Geometry: final body of the model. Coordinates: model frame, mm. Give positions to 0.01 mm unless a question says otherwise; leave off trailing zeros. Loops run counter-clockwise (first coordinate to the right, second up) from the corner with the lowest first, then second, coordinate; pieces in that order, holes last. Notation, with made-up numbers: (27, 72) -> (56, 72) arc R11 cw to (56, 93) -> close; hole circle Ø4 at (60, 57). An arc over 180 degrees is marked (long way). One line per item, written item: value. Start each with the question number.
from build123d import *
from OCP.BRepFilletAPI import BRepFilletAPI_MakeChamfer

# Parameters (mm, degrees)
BOSS_EXTRUDE1_DEPTH = 6
SKETCH2_W           = 9.8
SKETCH2_H           = 5.8
CUT_EXTRUDE1_DEPTH  = 6
SKETCH5_W           = 20
SKETCH5_H           = 236
CUT_EXTRUDE2_DEPTH  = 6
SKETCH6_W           = 10
SKETCH6_H           = 204
CUT_EXTRUDE3_DEPTH  = 20
SKETCH7_W           = 32
SKETCH7_H           = 236
CUT_EXTRUDE4_DEPTH  = 20
SKETCH8_W           = 248
SKETCH8_H           = 6
BOSS_EXTRUDE2_DEPTH = 5
SKETCH10_W          = 30
SKETCH10_H          = 204
BOSS_EXTRUDE3_DEPTH = 6
SKETCH11_W          = 21
SKETCH11_H          = 6
BOSS_EXTRUDE4_DEPTH = 30
CHAMFER1_SIZE       = 30
CHAMFER1_SIZE2      = 10.919107028
FILLET1_R           = 10


with BuildPart() as part:
    # Sketch1 → Boss-Extrude1 (new body)
    with BuildSketch(Plane(origin=(0, 0, 0), x_dir=(1, 0, 0), z_dir=(0, 1, 0))):
        Polygon((-150, 118), (-150, -118), (150, -118), (150, -102), (-98, -102), (-98, 102), (150, 102), (150, 118), align=None)
    extrude(amount=BOSS_EXTRUDE1_DEPTH)

    # Sketch2 → Cut-Extrude1 (cut)
    with BuildSketch(Plane(origin=(0, 6, 0), x_dir=(1, 0, 0), z_dir=(0, 1, 0))):
        with Locations((85, -110)):
            Rectangle(SKETCH2_W, SKETCH2_H)
        with Locations((115, -110)):
            Rectangle(SKETCH2_W, SKETCH2_H)
        with Locations((55, -110)):
            Rectangle(SKETCH2_W, SKETCH2_H)
        with Locations((25, -110)):
            Rectangle(SKETCH2_W, SKETCH2_H)
        with Locations((-5, -110)):
            Rectangle(SKETCH2_W, SKETCH2_H)
        with Locations((-35, -110)):
            Rectangle(SKETCH2_W, SKETCH2_H)
        with Locations((-65, -110)):
            Rectangle(SKETCH2_W, SKETCH2_H)
        with Locations((-95, -110)):
            Rectangle(SKETCH2_W, SKETCH2_H)
    cut_extrude1 = extrude(amount=-CUT_EXTRUDE1_DEPTH, mode=Mode.SUBTRACT)

    # Mirror1: Cut-Extrude1 across plane
    add(cut_extrude1.mirror(Plane.XY), mode=Mode.SUBTRACT)

    # Sketch5 → Cut-Extrude2 (cut)
    with BuildSketch(Plane(origin=(0, 6, 0), x_dir=(1, 0, 0), z_dir=(0, 1, 0))):
        with Locations((140, 0)):
            Rectangle(SKETCH5_W, SKETCH5_H)
    extrude(amount=-CUT_EXTRUDE2_DEPTH, mode=Mode.SUBTRACT)

    # Sketch6 → Cut-Extrude3 (cut)
    with BuildSketch(Plane(origin=(0, 6, 0), x_dir=(1, 0, 0), z_dir=(0, 1, 0))):
        with Locations((-103, 0)):
            Rectangle(SKETCH6_W, SKETCH6_H)
    extrude(amount=-CUT_EXTRUDE3_DEPTH, mode=Mode.SUBTRACT)

    # Sketch7 → Cut-Extrude4 (cut)
    with BuildSketch(Plane(origin=(0, 6, 0), x_dir=(1, 0, 0), z_dir=(0, 1, 0))):
        with Locations((-134, 0)):
            Rectangle(SKETCH7_W, SKETCH7_H)
    extrude(amount=-CUT_EXTRUDE4_DEPTH, mode=Mode.SUBTRACT)

    # Sketch8 → Boss-Extrude2 (add)
    with BuildSketch(Plane.XY.offset(118)):
        with Locations((6, 3)):
            Rectangle(SKETCH8_W, SKETCH8_H)
    boss_extrude2 = extrude(amount=BOSS_EXTRUDE2_DEPTH)

    # Mirror2: Boss-Extrude2 across plane
    add(boss_extrude2.mirror(Plane.XY))

    # Sketch10 → Boss-Extrude3 (add, through all)
    with BuildSketch(Plane(origin=(0, 6, 0), x_dir=(1, 0, 0), z_dir=(0, 1, 0))):
        with Locations((-93, 0)):
            Rectangle(SKETCH10_W, SKETCH10_H)
    extrude(amount=-BOSS_EXTRUDE3_DEPTH)

    # Sketch11 → Boss-Extrude4 (add)
    with BuildSketch(Plane(origin=(130, 0, 0), x_dir=(0, 0, -1), z_dir=(1, 0, 0))):
        with Locations((-112.5, 3)):
            Rectangle(SKETCH11_W, SKETCH11_H)
        with Locations((112.5, 3)):
            Rectangle(SKETCH11_W, SKETCH11_H)
    extrude(amount=BOSS_EXTRUDE4_DEPTH)

    # Chamfer1: one chamfer whose edges measure the first distance from different faces: ONE call of the kernel's chamfer builder (chamfer() names one face for all edges)
    chamfer1_edges_1 = [part.edges().sort_by_distance(p)[0] for p in [
        (160, 3, 102),
    ]]
    chamfer1_side_1 = [part.faces().sort_by_distance(p)[0] for p in [
        (41, 3, 102),
    ]]
    chamfer1_edges_2 = [part.edges().sort_by_distance(p)[0] for p in [
        (160, 3, -102),
    ]]
    chamfer1_side_2 = [part.faces().sort_by_distance(p)[0] for p in [
        (41, 3, -102),
    ]]
    chamfer1 = BRepFilletAPI_MakeChamfer(part.part.solid().wrapped)
    for e in chamfer1_edges_1:
        chamfer1.Add(CHAMFER1_SIZE, CHAMFER1_SIZE2, e.wrapped, chamfer1_side_1[0].wrapped)  # the first distance lies on this face
    for e in chamfer1_edges_2:
        chamfer1.Add(CHAMFER1_SIZE, CHAMFER1_SIZE2, e.wrapped, chamfer1_side_2[0].wrapped)  # the first distance lies on this face
    add(Compound.cast(chamfer1.Shape()), mode=Mode.REPLACE)

    # Fillet1
    fillet1_edges = [part.edges().sort_by_distance(p)[0] for p in [
        (160, 3, 112.919107028),
        (130, 3, 102),
        (160, 3, -112.919107028),
        (130, 3, -102),
    ]]
    fillet(fillet1_edges, radius=FILLET1_R)


solid = part.part
Item 1: Mould query, pull axis X, two halves, no side actions, for faces 1 (the face through (-60.1, 3, 110)), 2 (the face through (-83, 0, 1)), 3 (the face through (85, 3, 107.1)). Classes: pulls with the +X half, pulls with the -X half, needs draft (parallel to the pull), parting line crosses it, or undercut.
Item 2: Ray query, line 1 along Z through (x, y) = (-92, 4.55); line 2 along Z through (x, y) = (53.5, 3.95); line 3 along Z through (x, y) = (17.5, 2.3). Return the intervals inside material, ascending. Write a range as [from, to].
Item 3: Section B-B, the plane y = 2.15. State how many separate pieces and enclosed holes the cut face has, then the cut area to 3 significant figures.
Item 4: Section A-A, the plane x = 86. Output: boundary loops of the cut face in (y, z).
Item 5: Section C-C, the plane z = -76. Output: boundary loops of the cut face in (x, y), then the cut area to 3 significant figures.
Item 6: Pin query (flat end, axial travel): pin 1 (3 mm diameter, centred on y = 3.5, z = -109.5, fed in from +X); pin 2 (1.7 mm diameter, centred on y = 4.5, z = -111, fed in from +X); pin 3 (8 mm diameter, centred on x = -75, z = -71, fed in from +Y). Return the tip coordinate at first contact, or that it passes through.
Geometry check:
1. face 1: undercut
1. face 2: needs draft
1. face 3: undercut
2. line 1: z = [-123, -112.9], [-107.1, 107.1], [112.9, 123]
2. line 2: z = [-123, -112.9], [-107.1, -102], [102, 107.1], [112.9, 123]
2. line 3: z = [-123, -102], [102, 123]
3. separate pieces: 1
3. enclosed holes: 16
3. area: 18,600 mm2
4. outline: (0, -123) -> (6, -123) -> (6, -112.9) -> (0, -112.9) -> close; (0, -107.1) -> (6, -107.1) -> (6, -102) -> (0, -102) -> close; (0, 102) -> (6, 102) -> (6, 107.1) -> (0, 107.1) -> close; (0, 112.9) -> (6, 112.9) -> (6, 123) -> (0, 123) -> close
5. outline: (-118, 0) -> (-78, 0) -> (-78, 6) -> (-118, 6) -> close
5. area: 240 mm2
6. pin 1: stops at x = 154.52
6. pin 2: stops at x = 155.9
6. pin 3: stops at y = 6
